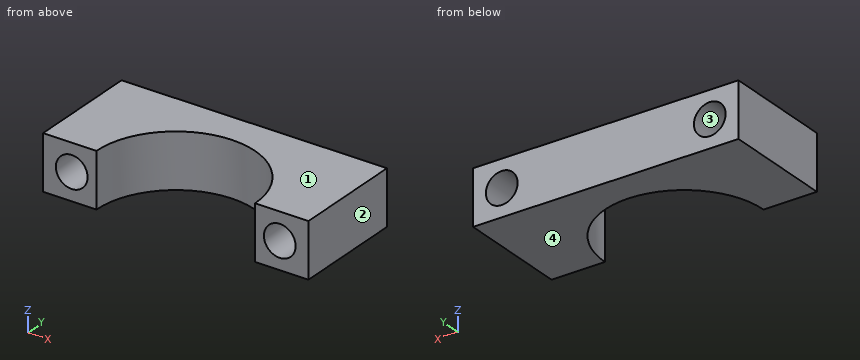
```python
from build123d import *

# Parameters (mm, degrees)
BOSS_EXTRUDE1_DEPTH = 2.75
SKETCH2_R           = 1.6
CUT_EXTRUDE1_DEPTH  = 18.742956349


with BuildPart() as part:
    # Sketch1 → Boss-Extrude1 (new, symmetric)
    with BuildSketch(Plane.XY):
        with BuildLine():
            Line((-13.4, 11.3), (13.4, 11.3))
            Line((13.4, 11.3), (13.4, 0))
            Line((13.4, 0), (8, 0))
            ThreePointArc((8, 0), (0, 8), (-8, 0))
            Line((-8, 0), (-13.4, 0))
            Line((-13.4, 0), (-13.4, 11.3))
        make_face()
    extrude(amount=BOSS_EXTRUDE1_DEPTH, both=True)

    # Sketch2 → Cut-Extrude1 (cut, through all)
    with BuildSketch(Plane.XZ):
        with Locations((-10.5, 0)):
            Circle(SKETCH2_R)
        with Locations((10.5, 0)):
            Circle(SKETCH2_R)
    extrude(amount=-CUT_EXTRUDE1_DEPTH, mode=Mode.SUBTRACT)


solid = part.part
```
Here's how the part is built. I have some questions about the finished solid (model axes, mm). Face numbers are marked on the shaded views. Give positions to 0.01 mm unless a question says otherwise; leave off trailing zeros. Loops run counter-clockwise (first coordinate to the right, second up) from the corner with the lowest first, then second, coordinate; pieces in that order, holes last. Notation, with made-up numbers: M -32.75,47 L -22.75,47 A17 cw -22.75,74 Z; hole C 9,80.25 d6. An arc over 180 degrees is marked long. Use one line per item in the form item = value. Start each with the question number.
Q1. If we section it at B-B (y = 3.5): Write out the boundary of the cut face in (x, z).
Q2. If we section it at D-D (y = 8.5): Write out the boundary of the cut face in (x, z).
Q3. If we section it at C-C (z = -0.5): Write out the boundary of the cut face in (x, y), then the cut area to 3 significant figures.
Q4. Thinking about a two-plate mould opening in Z: for the marked faces 1, 2, 3 and 4, which applies, +Z half, -Z half, draft (parallel to the pull), parting line (faces both ways), or undercut?
Q5. I need wall thicknesses on line 1 along X through (y, z) = (9.75, -0.1); line 2 along Z through (x, y) = (-10.5, 8.5); line 3 along X through (y, z) = (11.25, -1). Which ranges of each line are inside material? Lowest first, please.
Q6. Will these pins go through, and if not, where does the flat tip stop? pin 1 Ø3 at (x, z) = (3.5, 1.5) entering from -Y (3 decimals); pin 2 Ø1.5 at (x, z) = (5, 1.5) entering from -Y.
Q7. If we section it at A-A (x = 10.5): Write out the boundary of the cut face in (y, z), then the cut area to 3 significant figures.
Taken from the geometry:
q1.outline = M -13.4,-2.75 L -7.19,-2.75 L -7.19,2.75 L -13.4,2.75 Z; M 7.19,-2.75 L 13.4,-2.75 L 13.4,2.75 L 7.19,2.75 Z; hole C -10.5,0 d3.2; hole C 10.5,0 d3.2
q2.outline = M -13.4,-2.75 L 13.4,-2.75 L 13.4,2.75 L -13.4,2.75 Z; hole C -10.5,0 d3.2; hole C 10.5,0 d3.2
q3.outline = M -13.4,0 L -12.02,0 L -12.02,11.3 L -13.4,11.3 Z; M -8.98,0 L -8,0 A8 cw 8,0 L 8.98,0 L 8.98,11.3 L -8.98,11.3 Z; M 12.02,0 L 13.4,0 L 13.4,11.3 L 12.02,11.3 Z
q3.area = 134 mm^2
q4.face_1 = +Z half
q4.face_2 = draft
q4.face_3 = undercut
q4.face_4 = -Z half
q5.line_1 = -13.4 to -12.1, -8.9 to 8.9, 12.1 to 13.4
q5.line_2 = -2.75 to -1.6, 1.6 to 2.75
q5.line_3 = -13.4 to -11.75, -9.25 to 9.25, 11.75 to 13.4
q6.pin_1 = 6.245
q6.pin_2 = 5.56
q7.outline = M 0,-2.75 L 11.3,-2.75 L 11.3,-1.6 L 0,-1.6 Z; M 0,1.6 L 11.3,1.6 L 11.3,2.75 L 0,2.75 Z
q7.area = 26.0 mm^2
